Autodesk Inventor part; units mm, degrees
ref_plane "YZ Plane" through (0, 0, 0) normal (1, 0, 0) x (0, 1, 0)
ref_plane "XZ Plane" through (0, 0, 0) normal (0, 1, 0) x (-1, 0, 0)
ref_plane "XY Plane" through (0, 0, 0) normal (0, 0, 1) x (1, 0, 0)
sketch "Sketch1" plane through (0, 0, 0) normal (0, 1, 0) x (-1, 0, 0)
  circle A0 centre (0, 0) radius 215
  circle A1 centre (0, 0) radius 315
  line L0 (0, 0) -> (-315, 0)
  line L1 (0, 0) -> (-222.7386, 222.7386)
  line L2 (0, 0) -> (-313.8013, -27.4541)
  line L3 (0, 0) -> (-241.304, 202.4781)
  circle A2 centre (0, 0) radius 230
  circle A3 centre (0, 0) radius 300
  point P0 (-152.028, 152.028)
  point P1 (-215, 0)
  point P2 (-212.132, 212.132)
  point P3 (-229.8133, 192.8363)
  point P4 (-298.8584, -26.1467)
  point P5 (-300, 0)
  point P6 (-230, 0)
  point P7 (-229.1248, -20.0458)
  point P8 (-214.1819, -18.7385)
  point P9 (-164.6996, 138.1993)
  point P10 (-176.1902, 147.8412)
  point P11 (-162.6346, 162.6346)
  dimension "d1" = 430
  dimension "d2" = 45
  dimension "d31" = 100
  dimension "d47" = 5
  dimension "d48" = 5
  dimension "d49" = 15
  dimension "d50" = 15
extrude "Extrusion1" add sketch "Sketch1" along normal blind 5 contours L2 A2 L0 A0 | A0 L0 A2 L3 | A2 L3 A3 L1 | A2 L0 A3 L3 | L2 A1 L0 A3 | A3 L0 A1 L3
sketch "Sketch2" plane through (0, 0, 0) normal (0, 1, 0) x (1, 0, 0)
  circle A0 centre (0, 0) radius 205
  circle A1 centre (0, 0) radius 215
  circle A2 centre (0, 0) radius 315
  circle A3 centre (0, 0) radius 325
  line L0 (0, 0) -> (259.5565, -195.5899)
  line L1 (0, 0) -> (275.6156, -172.2238)
  line L2 (0, 0) -> (317.898, -67.5713)
  line L3 (0, 0) -> (322.5775, -39.6075)
  line L4 (300, 0) -> (230, 0)
  point P0 (315, 0)
  point P1 (215, 0)
  point P2 (312.652, -38.3888)
  point P3 (308.1165, -65.4922)
  point P4 (213.3974, -26.2019)
  point P5 (203.472, -24.9832)
  point P6 (200.5203, -42.6219)
  point P7 (210.3017, -44.701)
  point P8 (267.1352, -166.9246)
  point P9 (251.5702, -189.5717)
  point P10 (182.3303, -113.9326)
  point P11 (173.8499, -108.6334)
  point P12 (163.7203, -123.3721)
  point P13 (171.7066, -129.3902)
  dimension "d5" = 410
  dimension "d6" = 10
  dimension "d7" = 100
  dimension "d8" = 10
  dimension "d9" = 7
  dimension "d10" = 5
  dimension "d11" = 20
  dimension "d12" = 5
extrude "Extrusion2" add sketch "Sketch2" along normal blind 30 contours A0 L1 A1 L0 | L3 A1 L2 A0 | A2 L1 A3 L0 | L3 A3 L2 A2
chamfer "Chamfer1" distance 10 angle 45 4 edges at (177.1871, 30, 121.7773) (259.5997, 30, 178.418) (212.0514, 30, 35.4852) (310.68, 30, 51.99)
sketch "Sketch3" plane through (0, 5, 0) normal (0, 1, 0) x (1, 0, 0)
  circle A0 centre (0, 0) radius 235
  circle A1 centre (0, 0) radius 285
  arc A2 (251.5702, -189.5717) -> (267.1352, -166.9246) centre (0, 0) ccw
  arc A3 (308.1165, -65.4922) -> (312.652, -38.3888) centre (0, 0) ccw
  arc A4 (241.304, -202.4781) -> (251.5702, -189.5717) centre (0, 0) ccw
  line L0 (300, 0) -> (230, 0)
  arc A5 (213.3974, -26.2019) -> (214.1819, 18.7385) centre (0, 0) ccw
  line L1 (162.6346, -162.6346) -> (212.132, -212.132)
  line L2 (166.1701, -166.1701) -> (201.5254, -201.5254)
  arc A6 (312.652, -38.3888) -> (313.8013, 27.4541) centre (0, 0) ccw
  arc A7 (267.1352, -166.9246) -> (308.1165, -65.4922) centre (0, 0) ccw
  arc A8 (171.7066, -129.3902) -> (182.3303, -113.9326) centre (0, 0) ccw
  arc A9 (164.6996, -138.1993) -> (171.7066, -129.3902) centre (0, 0) ccw
  arc A10 (210.3017, -44.701) -> (213.3974, -26.2019) centre (0, 0) ccw
  arc A11 (182.3303, -113.9326) -> (210.3017, -44.701) centre (0, 0) ccw
  line L3 (235, 0) -> (284.6303, 0)
  line L4 (284.8245, -10) -> (234.7871, -10)
  line L5 (208.4724, -194.3303) -> (173.0906, -158.9485)
  line L6 (229.8133, -192.8363) -> (241.304, -202.4781)
  line L7 (313.8013, 27.4541) -> (298.8584, 26.1467)
  arc A12 (300, 0) -> (298.8584, 26.1467) centre (0, 0) ccw
  arc A13 (230, 0) -> (229.1248, 20.0458) centre (0, 0) ccw
  line L8 (229.1248, 20.0458) -> (214.1819, 18.7385)
  line L9 (164.6996, -138.1993) -> (176.1902, -147.8412)
  arc A14 (162.6346, -162.6346) -> (176.1902, -147.8412) centre (0, 0) ccw
  arc A15 (212.132, -212.132) -> (229.8133, -192.8363) centre (0, 0) ccw
  point P0 (235, 0)
  point P1 (172.3223, -159.7812)
  point P2 (208.9866, -193.7772)
  point P3 (166.1701, -166.1701)
  point P4 (201.5254, -201.5254)
  point P5 (285, 0)
  point P6 (235, 0)
  point P7 (183.8478, -183.8478)
  point P8 (187.3833, -187.3833)
  dimension "d18" = 470
  dimension "d22" = 0
  dimension "d32" = 50
  dimension "d33" = 10
  dimension "d34" = 0
  dimension "d43" = 10
extrude "Extrusion3" add sketch "Sketch3" along normal blind 30 contours L0 A1 L4 A0 | A0 L5 A1 L1
chamfer "Chamfer3" distance 9 angle 45 2 edges at (259.8058, 35, 10) (190.7815, 35, 176.6394)
fillet "Fillet1" radius 10 6 edges at (259.8058, 26, 10) (310.68, 20.0005, 51.99) (259.5997, 20.0005, 178.418) (177.1871, 20.0005, 121.7773) (212.0514, 20.0005, 35.4852) (190.7815, 26, 176.6394)
sketch "Sketch4" plane through (0, 5, 0) normal (0, 1, 0) x (1, 0, 0)
  arc A0 (201.5254, -201.5254) -> (208.4724, -194.3303) centre (0, 0) ccw
  line L0 (201.5254, -201.5254) -> (212.132, -212.132)
  arc A1 (241.304, -202.4781) -> (251.5702, -189.5717) centre (0, 0) ccw
  arc A2 (251.5702, -189.5717) -> (267.1352, -166.9246) centre (0, 0) ccw
  arc A3 (267.1352, -166.9246) -> (308.1165, -65.4922) centre (0, 0) ccw
  arc A4 (308.1165, -65.4922) -> (312.652, -38.3888) centre (0, 0) ccw
  arc A5 (312.652, -38.3888) -> (313.8013, 27.4541) centre (0, 0) ccw
  line L1 (300, 0) -> (285, 0)
  arc A6 (284.8245, -10) -> (285, 0) centre (0, 0) ccw
  line L2 (284.8245, -10) -> (234.7871, -10)
  arc A7 (234.7871, -10) -> (235, 0) centre (0, 0) ccw
  line L3 (235, 0) -> (230, 0)
  arc A8 (213.3974, -26.2019) -> (214.1819, 18.7385) centre (0, 0) ccw
  arc A9 (210.3017, -44.701) -> (213.3974, -26.2019) centre (0, 0) ccw
  arc A10 (182.3303, -113.9326) -> (210.3017, -44.701) centre (0, 0) ccw
  arc A11 (171.7066, -129.3902) -> (182.3303, -113.9326) centre (0, 0) ccw
  arc A12 (164.6996, -138.1993) -> (171.7066, -129.3902) centre (0, 0) ccw
  line L4 (162.6346, -162.6346) -> (166.1701, -166.1701)
  arc A13 (166.1701, -166.1701) -> (173.0906, -158.9485) centre (0, 0) ccw
  line L5 (234.7871, -10) -> (214.7673, -10)
  arc A14 (213.3974, -26.2019) -> (214.1819, 18.7385) centre (0, 0) ccw
  line L6 (284.8245, -10) -> (314.8412, -10)
  line L7 (171.8681, -160.2696) -> (157.241, -146.6296)
  line L8 (208.4358, -194.3695) -> (230.3764, -214.8295)
  arc A15 (241.304, -202.4781) -> (251.5702, -189.5717) centre (0, 0) ccw
  line L9 (173.0906, -158.9485) -> (208.4724, -194.3303)
  arc A16 (230, 0) -> (229.1248, 20.0458) centre (0, 0) ccw
  line L10 (229.1248, 20.0458) -> (214.1819, 18.7385)
  line L11 (164.6996, -138.1993) -> (176.1902, -147.8412)
  arc A17 (162.6346, -162.6346) -> (176.1902, -147.8412) centre (0, 0) ccw
  arc A18 (212.132, -212.132) -> (229.8133, -192.8363) centre (0, 0) ccw
  line L12 (229.8133, -192.8363) -> (241.304, -202.4781)
  line L13 (313.8013, 27.4541) -> (298.8584, 26.1467)
  arc A19 (300, 0) -> (298.8584, 26.1467) centre (0, 0) ccw
  point P0 (222.7386, -222.7386)
  point P1 (215, 0)
  dimension "d39" = 43
sketch "Sketch5" plane through (0, 5, 0) normal (0, 1, 0) x (1, 0, 0)
  arc A0 (234.7871, -10) -> (235, 0) centre (0, 0) ccw
  line L0 (235, 0) -> (230, 0)
  arc A1 (213.3974, -26.2019) -> (214.1819, 18.7385) centre (0, 0) ccw
  arc A2 (210.3017, -44.701) -> (213.3974, -26.2019) centre (0, 0) ccw
  arc A3 (182.3303, -113.9326) -> (210.3017, -44.701) centre (0, 0) ccw
  arc A4 (171.7066, -129.3902) -> (182.3303, -113.9326) centre (0, 0) ccw
  arc A5 (164.6996, -138.1993) -> (171.7066, -129.3902) centre (0, 0) ccw
  line L1 (162.6346, -162.6346) -> (166.1701, -166.1701)
  arc A6 (166.1701, -166.1701) -> (173.0906, -158.9485) centre (0, 0) ccw
  line L2 (173.0906, -158.9485) -> (208.4724, -194.3303)
  arc A7 (201.5254, -201.5254) -> (208.4724, -194.3303) centre (0, 0) ccw
  line L3 (201.5254, -201.5254) -> (212.132, -212.132)
  arc A8 (241.304, -202.4781) -> (251.5702, -189.5717) centre (0, 0) ccw
  arc A9 (251.5702, -189.5717) -> (267.1352, -166.9246) centre (0, 0) ccw
  arc A10 (267.1352, -166.9246) -> (308.1165, -65.4922) centre (0, 0) ccw
  arc A11 (308.1165, -65.4922) -> (312.652, -38.3888) centre (0, 0) ccw
  arc A12 (312.652, -38.3888) -> (313.8013, 27.4541) centre (0, 0) ccw
  line L4 (300, 0) -> (285, 0)
  arc A13 (284.8245, -10) -> (285, 0) centre (0, 0) ccw
  line L5 (284.8245, -10) -> (234.7871, -10)
  line L6 (222.7386, -222.7386) -> (0, 0) construction
  line L7 (0, 0) -> (315, 0) construction
  circle A14 centre (0, 0) radius 215
  circle A15 centre (0, 0) radius 315
  arc A16 (230, 0) -> (229.1248, 20.0458) centre (0, 0) ccw
  line L8 (229.1248, 20.0458) -> (214.1819, 18.7385)
  line L9 (164.6996, -138.1993) -> (176.1902, -147.8412)
  arc A17 (162.6346, -162.6346) -> (176.1902, -147.8412) centre (0, 0) ccw
  arc A18 (212.132, -212.132) -> (229.8133, -192.8363) centre (0, 0) ccw
  line L10 (229.8133, -192.8363) -> (241.304, -202.4781)
  line L11 (313.8013, 27.4541) -> (298.8584, 26.1467)
  arc A19 (300, 0) -> (298.8584, 26.1467) centre (0, 0) ccw
  dimension "d44" = 45
  dimension "d45" = 630
  dimension "d46" = 430
properties part number "MC Plate" material "MDF Medium Density Fiberboard"
Build history of the part. All positions in model axes, mm. A direction names the side the tool comes from. Coordinates: 2 decimals unless noted, no trailing zeros. Order: outer loops, then holes, each group sorted by start corner. A loop starts at its lowest first (then second) coordinate and runs counter-clockwise, first axis right, second up. Notation, with made-up numbers: M -36,76 L -8,76 A18 cw -8,90 Z; hole C -13.75,70 d4. An arc over 180 degrees is marked long. One line per question, with ' | ' between items. Start each with the question number.
Q1. Flat gauge pins, fed straight in: pin 1 Ø10.5 at (x, y) = (260.5, 23.5) entering from -Z; pin 2 Ø5 at (x, z) = (170.5, 114) entering from +Y; pin 3 Ø8 at (y, z) = (22.5, 126) entering from +X. Where does each tip first touch, or does it go through?
Q2. Saw through at A-A (y = 13). List the corners of the cut face in (x, z).
Q3. Saw through at C-C (x = 225). List the corners of the cut face in (y, z).
Q4. Saw through at B-B (z = 18). List the corners of the cut face in (x, y), then the cut area to 3 significant figures.
Q5. Probe L1, parallel to Y at x = 181.5, z = 148; L2, parallel to Z at x = 278, y = 21.5; L3, parallel to X at y = 14, z = 180. List the from-to ranges inside material, lowest first. Write a range as from..to.
Q6. 3-axis set-ups, long thin cutter, end or side, ignore diameter. For faces 4 (the face through (212.073, 10.353, 35.356)), 5 (the face through (229.775, 2.465, -10.173)), 6 (the face through (205.343, 11.457, 43.647)): which of +Z, -Z, +X, -X, +Y, -Y reach the whole face in a straight line?
Q7. Two-plate mould, pull along X, no slides. Class faces 1 (the face through (191.03, 13.31, 176.89)), 2 (the face through (267.95, 14.79, 183.92)), 3 (the face through (234.95, 19.79, 4.93)): +X half, -X half, draft (parallel to the pull), parting line (faces both ways), or undercut.
Check values:
1) pin 1: stops at z = 0 | pin 2: stops at y = 30 | pin 3: stops at x = 175.33
2) outline: M 163.72,123.37 A205 cw 173.85,108.63 L 182.33,113.93 A215 ccw 171.71,129.39 Z; M 166.17,166.17 A235 cw 173.09,158.95 L 208.47,194.33 A285 ccw 201.53,201.53 Z; M 200.52,42.62 A205 cw 203.47,24.98 L 213.4,26.2 A215 ccw 210.3,44.7 Z; M 234.79,10 A235 cw 235,0 L 285,0 A285 ccw 284.82,10 Z; M 251.57,189.57 A315 cw 267.14,166.92 L 275.62,172.22 A325 ccw 259.56,195.59 Z; M 308.12,65.49 A315 cw 312.65,38.39 L 322.58,39.61 A325 ccw 317.9,67.57 Z
3) outline: M 0,-19.68 L 5,-19.68 L 5,198.43 L 0,198.43 Z
4) outline: M 214.25,0 L 314.49,0 L 314.49,5 L 214.25,5 Z | area: 501 mm2
5) L1: y = 0..5 | L2: z = 0..10 | L3: x = 180..194.14, 258.51..270.6
6) face 4: +Z, +Y | face 5: -Z, +Y, -Y | face 6: -X, +Y, -Y
7) face 1: undercut | face 2: +X half | face 3: -X half
